from build123d import *

# Parameters (mm, degrees)
F1_DEPTH = 8
F2_R     = 4.5
F3_DEPTH = 8
F6_R     = 1
F8_W     = 3
F8_H     = 18.55


with BuildPart() as f1:
    # F0 (on Front) → F1 (new body)
    with BuildSketch(Plane.XZ):
        with BuildLine():
            Line((-39.575, 28.175), (-39.575, 0))
            Line((-39.575, 0), (-39.575, -28.175))
            add(Edge.make_bspline(
                [(-39.575, -28.175), (-39.8652448061, -32.0825006212), (-35.9525292205, -38.4365629841), (-22.6949341127, -34.0786260822), (-8.920869255, -39.156793634), (-2.73677378, -39.4421363997), (0, -39.575)],
                knots=[0, 0, 0, 0, 0.2247670207, 0.4893991001, 0.7773525509, 1, 1, 1, 1], degree=3))
            add(Edge.make_bspline(
                [(39.575, -28.175), (39.8652448061, -32.0825006212), (35.9525292205, -38.4365629841), (22.6949341127, -34.0786260822), (8.920869255, -39.156793634), (2.73677378, -39.4421363997), (0, -39.575)],
                knots=[0, 0, 0, 0, 0.2247670207, 0.4893991001, 0.7773525509, 1, 1, 1, 1], degree=3))
            Line((39.575, -28.175), (39.575, 0))
            Line((39.575, 0), (39.575, 28.175))
            add(Edge.make_bspline(
                [(39.575, 28.175), (39.8652448061, 32.0825006212), (35.9525292205, 38.4365629841), (22.6949341127, 34.0786260822), (8.920869255, 39.156793634), (2.73677378, 39.4421363997), (0, 39.575)],
                knots=[0, 0, 0, 0, 0.2247670207, 0.4893991001, 0.7773525509, 1, 1, 1, 1], degree=3))
            add(Edge.make_bspline(
                [(-39.575, 28.175), (-39.8652448061, 32.0825006212), (-35.9525292205, 38.4365629841), (-22.6949341127, 34.0786260822), (-8.920869255, 39.156793634), (-2.73677378, 39.4421363997), (0, 39.575)],
                knots=[0, 0, 0, 0, 0.2247670207, 0.4893991001, 0.7773525509, 1, 1, 1, 1], degree=3))
        make_face()
    extrude(amount=F1_DEPTH)

    # F2 (on face) → F3 (cut, through all)
    with BuildSketch(Plane.XZ.offset(8)):
        with Locations((-31.6271925499, 28.6181603254)):
            Circle(F2_R)
        with Locations((-31.4327607315, -28.8315792456)):
            Circle(F2_R)
        with Locations((31.5314427808, -28.7236231203)):
            Circle(F2_R)
        with Locations((31.1694185133, 29.1160738862)):
            Circle(F2_R)
    extrude(amount=-F3_DEPTH, mode=Mode.SUBTRACT)

    # F7: sweep along a path in F5
    with BuildLine(Plane.XZ.offset(8)) as f7_path:
        CenterArc((0, 0), 32.875, 0, 360)
    # F6 (on Top) → F7 (sweep, cut)
    with BuildSketch(Plane.XY):
        with Locations((32.875, -8)):
            Circle(F6_R)
    sweep(path=f7_path.line, mode=Mode.SUBTRACT)

    # F9: sweep along a path in F4
    with BuildLine(Plane(origin=(0, 0, 0), x_dir=(-1, 0, 0), z_dir=(0, 1, 0))) as f9_path:
        CenterArc((0, 0), 34.95, 0, 360)
    # F8 (on Top) → F9 (sweep)
    with BuildSketch(Plane.XY):
        with Locations((34.95, 9.275)):
            Rectangle(F8_W, F8_H)
    sweep(path=f9_path.line)


solid = f1.part
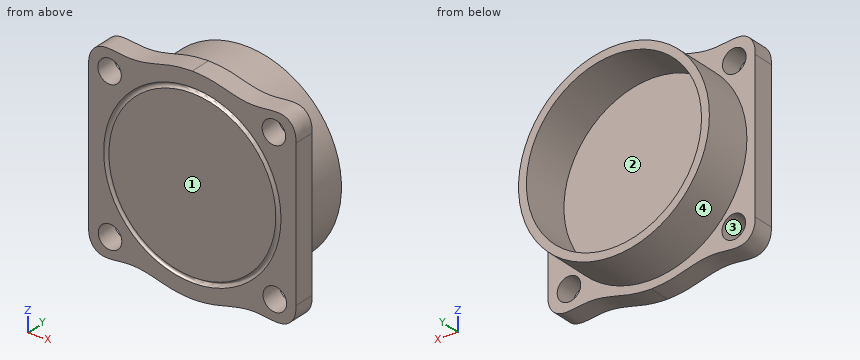
CAD build for the part. Positions are in the model's coordinates, mm. Face numbers are marked on the shaded views. A direction names the side the tool comes from. Coordinates: 2 decimals unless noted, no trailing zeros. Loops run counter-clockwise (first coordinate to the right, second up) from the corner with the lowest first, then second, coordinate; pieces in that order, holes last. Notation, with made-up numbers: (23, -33) - (75, -33) arc R18 ccw to (75, -1) - close; hole circle Ø11 at (67.5, -10.75). An arc over 180 degrees is marked (long way). Write item = value, one per line. Start each with the question number.
Q1. Pull direction Z, two halves, no side cores. Call the marked faces 3 and 4: pulls with the +Z half, pulls with the -Z half, needs draft (parallel to the pull), parting line crosses it, or undercut.
Q2. Flat gauge pins, fed straight in: pin 1 Ø5 at (x, y) = (-21, 15.5) entering from +Z; pin 2 Ø3 at (x, y) = (-17, 6.5) entering from +Z; pin 3 Ø1 at (y, z) = (-1.5, -26) entering from -X (3 decimals). Where does each tip first touch, or does it go through?
Q3. Which spindle directions (+Z, -Z, +X, -X, +Y, -Y) get a long thin tool onto all of the face, cutting with end or side? Do the marked faces 1 and 2. Say none if no direction does.
Q4. Cut at A-A, the plane y = 16.5. List the corners of the cut face in (x, z), then the cut area to 3 significant figures.
Q5. Cut at B-B, the plane x = -30. Give the number of separate pieces and of enclosed holes in the cut face, then the cut area to 3 significant figures.
Q6. Drill centre lines: L1, parallel to Z at x = 0, y = 10.25; L2, parallel to Y at x = -9.5, z = -30; L3, parallel to Z at x = -26, y = 4.75. Where is each one in solid material? Low to high.
Computed:
q1.face_3 = undercut
q1.face_4 = parting line crosses it
q2.pin_1 = 31.41
q2.pin_2 = 32.99
q2.pin_3 = -39.575
q3.face_1 = +Z, -Z, +X, -X, -Y
q3.face_2 = +Y
q4.outline = circle Ø72.9 at (0, 0); hole circle Ø66.9 at (0, 0)
q4.area = 659 mm²
q5.separate_pieces = 3
q5.enclosed_holes = 0
q5.area = 657 mm²
q6.L1 = -36.45 to -33.45, 33.45 to 36.45
q6.L2 = -8 to 0
q6.L3 = -25.55 to -21.05, 21.05 to 25.55
